```python
from build123d import *

# Parameters (mm, degrees)
F1_DEPTH = 25.4


with BuildPart() as f1:
    # F0 (on Right) → F1 (new body)
    with BuildSketch(Plane.YZ):
        with BuildLine():
            Line((3.81, -6.35), (12.7, -6.35))
            Line((12.7, -6.35), (12.7, 6.35))
            Line((12.7, 6.35), (-12.7, 6.35))
            Line((-12.7, 6.35), (-12.7, -6.35))
            Line((-12.7, -6.35), (-3.81, -6.35))
            ThreePointArc((-3.81, -6.35), (0, -5.08), (3.81, -6.35))
        make_face()
        with BuildLine():
            Line((12.7, -22.86), (12.7, -6.35))
            Line((12.7, -6.35), (3.81, -6.35))
            ThreePointArc((3.81, -6.35), (5.679613, -8.590194), (6.35, -11.43))
            ThreePointArc((6.35, -11.43), (-2.839806, -17.109613), (-3.81, -6.35))
            Line((-3.81, -6.35), (-12.7, -6.35))
            Line((-12.7, -6.35), (-12.7, -22.86))
            Line((-12.7, -22.86), (12.7, -22.86))
        make_face()
    extrude(amount=F1_DEPTH)


solid = f1.part
```
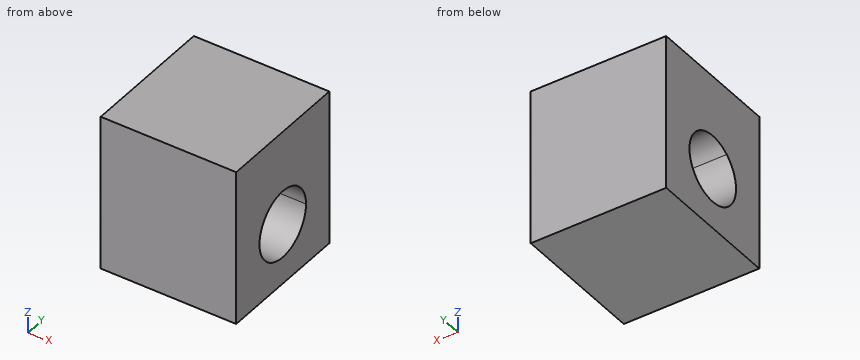
Design review of the part built by this model. Coordinates are the model's own, in mm. Coordinates: 2 decimals unless noted, no trailing zeros. Write each loop counter-clockwise with the first axis right and the second up, starting at its lowest first coordinate (ties: lowest second). Pieces come first, ordered by that corner, then holes. Notation, with made-up numbers: M 73,26.5 L 126,26.5 A20 cw 126,59.5 Z; hole C 76,-28.5 d10. An arc over 180 degrees is marked long. Answer as a JSON object with one key per item and string values.
Item 1: Add section B-B, the plane x = 9.25. Give the boundary of the cut face in (y, z), and give its area (3 significant figures).
Outcome:
{"outline": "M -12.7,-22.86 L 12.7,-22.86 L 12.7,6.35 L -12.7,6.35 Z; hole M 3.81,-6.35 A6.35 ccw long 6.35,-11.43 A6.35 ccw Z", "area": "615 mm²"}
Item 2: Add section C-C, the plane z = -10.5. Give the boundary of the cut face in (x, y), and give its area (3 significant figures).
Outcome:
{"outline": "M 0,-12.7 L 25.4,-12.7 L 25.4,-6.28 L 0,-6.28 Z; M 0,6.28 L 25.4,6.28 L 25.4,12.7 L 0,12.7 Z", "area": "326 mm²"}
Item 3: Insertion check: pin 1 Ø2 at (y, z) = (1, -15.5) entering from -X. The pin has a flat end and moves straight along its axis. Give the tip position at first contact, or say it passes through.
Outcome:
{"pin 1": "through"}
Item 4: Add section A-A, the plane y = 0. Give the boundary of the cut face in (x, z).
Outcome:
{"outline": "M 0,-22.86 L 25.4,-22.86 L 25.4,-17.78 L 0,-17.78 Z; M 0,-5.08 L 25.4,-5.08 L 25.4,6.35 L 0,6.35 Z"}
Item 5: Wall thickness on probe 1 along Y at (x, z) = (11.5, -11.43); probe 2 along Z at (x, y) = (5.75, 0); probe 3 along Z at (x, y) = (14.75, 2.5): over which ranges is each line inside the solid? List them lowest first.
Outcome:
{"probe 1": "-12.7 to -6.35, 6.35 to 12.7", "probe 2": "-22.86 to -17.78, -5.08 to 6.35", "probe 3": "-22.86 to -17.27, -5.59 to 6.35"}
